Input: part model. Units: mm. Frame: model coordinates. Face numbers are marked on the shaded views. A direction names the side the tool comes from. Coordinates: 2 decimals unless noted, no trailing zeros. Order: outer loops, then holes, each group sorted by start corner. A loop starts at its lowest first (then second) coordinate and runs counter-clockwise, first axis right, second up. Notation, with made-up numbers: (52.25, -11.5) - (68.25, -11.5) arc R35 ccw to (68.25, 26.5) - close; hole circle Ø11 at (87.25, 61.25). An arc over 180 degrees is marked (long way). One line per question, with ' | ' between items.
from build123d import *

# Parameters (mm, degrees)
SKETCH1_R           = 30.988
BOSS_EXTRUDE1_DEPTH = 147.32
SKETCH3_R           = 10.16
FILLET3_R           = 7.62
SKETCH8_R           = 10.16
BOSS_EXTRUDE2_DEPTH = 12.7
FILLET4_R           = 12.7


with BuildPart() as part:
    # Sketch1 → Boss-Extrude1 (new body)
    with BuildSketch(Plane(origin=(0, 0, 0), x_dir=(1, 0, 0), z_dir=(0, 1, 0))):
        with Locations(Location((0, 0, 0), (0, 0, 270))):
            Circle(SKETCH1_R)
    extrude(amount=BOSS_EXTRUDE1_DEPTH)

    # Sketch3 → section 1 of loft2
    with BuildSketch(Plane(origin=(0, 180.34, 0), x_dir=(-1, 0, 0), z_dir=(0, -1, 0)), mode=Mode.PRIVATE) as loft2_s1:
        Circle(SKETCH3_R)
    # loft up to a face of the part (loft2)
    loft([Face(Wire([part.edges().sort_by_distance((22.589279827, 147.32, -21.212745719))[0]])), loft2_s1.sketch])

    # Fillet3
    fillet3_edges = [part.edges().sort_by_distance(p)[0] for p in [
        (0, 147.32, -30.988),
    ]]
    fillet(fillet3_edges, radius=FILLET3_R)

    # Sketch8 → Boss-Extrude2 (add)
    with BuildSketch(Plane(origin=(0, 180.34, 0), x_dir=(1, 0, 0), z_dir=(0, 1, 0))):
        with Locations(Location((0, 0, 0), (0, 0, 270))):
            Circle(SKETCH8_R)
    extrude(amount=BOSS_EXTRUDE2_DEPTH)

    # Fillet4
    fillet4_edges = [part.edges().sort_by_distance(p)[0] for p in [
        (0, 0, -30.988),
    ]]
    fillet(fillet4_edges, radius=FILLET4_R)


solid = part.part
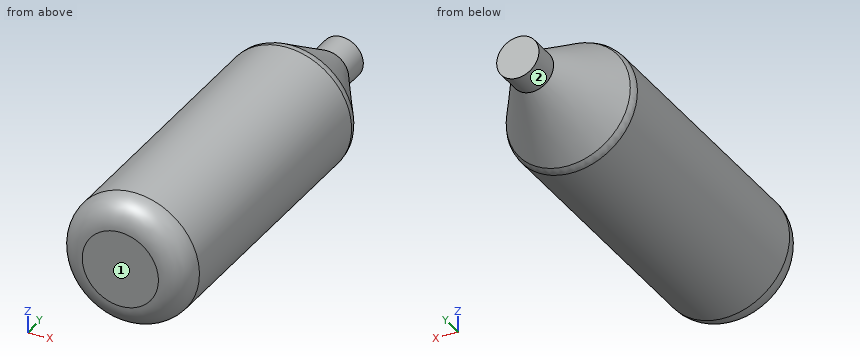
Item 1: Ray query, line 1 (X direction, y = 85, z = 0); line 2 (X direction, y = 52, z = 8.5); line 3 (Z direction, x = 16.5, y = 68). Return the intervals inside material, ascending.
Data:
line 1: -30.99 to 30.99 | line 2: -29.8 to 29.8 | line 3: -26.23 to 26.23
Item 2: Section B-B on y = 155. Return the cut outline in (x, z).
Data:
outline: circle Ø52.29 at (0, 0)
Item 3: Contact query for flat-ended pins moving along their axis: P1, Ø2, axis at y = 36, z = 20, coming from the -X side; P2, Ø12, axis at x = -20.5, y = 75.5, coming from the +Z side; P3, Ø6, axis at x = -3, y = 144.5, coming from the +Z side; P4, Ø10, axis at x = 17.5, y = 69, coming from the +Z side (3 decimals). Output: stop coordinate, or through.
Data:
P1: x = -24.48 | P2: z = 27.39 | P3: z = 30.99 | P4: z = 28.355
Item 4: Section A-A on y = 51. Return the cut outline in (x, z), and give its area (3 significant figures).
Data:
outline: circle Ø61.98 at (0, 0) | area: 3,020 mm^2
Item 5: Access query for the marked faces 1 and 2. Directions: +Z, -Z, +X, -X, +Y, -Y. A direction counts if a zero-diameter tool reaches every point of the face in a straight line with its end or side. Return the directions, or none.
Data:
face 1: +Z, -Z, +X, -X, -Y | face 2: +Y
